Source: CAD feature listing. Evaluate the final solid. Frame: model axes, mm. Face numbers are marked on the shaded views. A direction names the side the tool comes from. Give positions to 0.01 mm unless a question says otherwise; leave off trailing zeros. Order: outer loops, then holes, each group sorted by start corner. A loop starts at its lowest first (then second) coordinate and runs counter-clockwise, first axis right, second up. Notation, with made-up numbers: M 48,60.25 L 63,60.25 A25 cw 63,89.25 Z; hole C 65.25,-38.75 d11. An arc over 180 degrees is marked long. Answer in a Markdown table with one row per item. Add a question column.
(1) Pin query (flat end, axial travel): P1, Ø1.5, axis at x = 76.5, z = -47.5, coming from the +Y side; P2, Ø22.5, axis at x = 24.5, y = 1.5, coming from the +Z side; P3, Ø10, axis at y = 1, z = -11.5, coming from the +X side. Return the tip coordinate at first contact, or that it passes through.
(2) Section query C-C, the plane z = -19.5. Return loops of the section in (x, y), plus the area to 3 significant figures.
(3) Section query B-B, the plane x = -25.5. Return loops of the section in (y, z).
(4) Material intervals for line 1 along Z through (x, y) = (7, 19.4); line 2 along X through (y, z) = (19.45, -47); line 3 along Z through (x, y) = (-53, 16), sorted ascending.
(5) Set-up query: the marked faces 1 and 2. Return all of +Z, -Z, +X, -X, +Y, -Y with unobstructed straight access to the full face (end or side cutting, diameter ignored); none if empty.
(6) Section query A-A, the plane y = -16.5. Return loops of the section in (x, z).
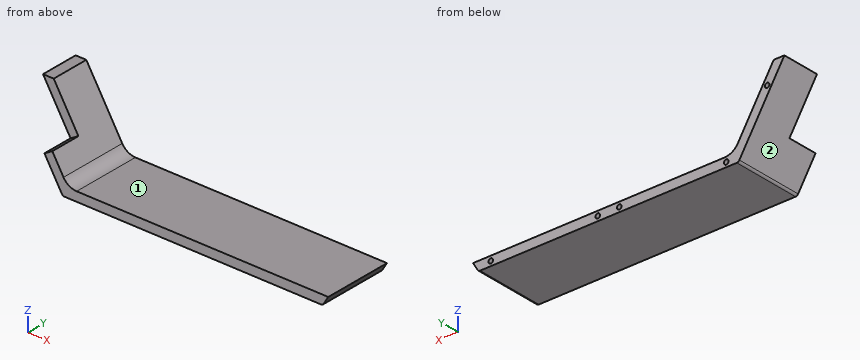
from build123d import *

# Parameters (mm, degrees)
BOSS_EXTRUDE1_DEPTH = 22.5
SKETCH2_R           = 1.5
CUT_EXTRUDE1_DEPTH  = 5
FILLET1_R           = 2
SKETCH3_W           = 35
SKETCH3_H           = 20
CUT_EXTRUDE2_DEPTH  = 10
SKETCH6_W           = 44
SKETCH6_H           = 45
CUT_EXTRUDE3_DEPTH  = 128.401923062
FILLET2_R           = 10


with BuildPart() as part:
    # Sketch1 → Boss-Extrude1 (new, symmetric)
    with BuildSketch(Plane(origin=(0, 0, 0), x_dir=(1, 0, 0), z_dir=(0, 1, 0))):
        Polygon((-115, 0), (-85, 50), (85, 50), (115, 0), (108, 0), (81.6, 44), (-81.6, 44), (-108, 0), align=None)
    extrude(amount=BOSS_EXTRUDE1_DEPTH, both=True)

    # Sketch2 → Cut-Extrude1 (cut)
    with BuildSketch(Plane(origin=(0, 22.5, 0), x_dir=(1, 0, 0), z_dir=(0, 1, 0))):
        with Locations(Location((-103.701428863, 13, 0), (0, 0, 270))):
            Circle(SKETCH2_R)
        with Locations(Location((-77, 47, 0), (0, 0, 270))):
            Circle(SKETCH2_R)
        with Locations(Location((-7, 47, 0), (0, 0, 270))):
            Circle(SKETCH2_R)
        with Locations(Location((7, 47, 0), (0, 0, 90))):
            Circle(SKETCH2_R)
        with Locations(Location((77, 47, 0), (0, 0, 90))):
            Circle(SKETCH2_R)
        with Locations(Location((103.701428863, 13, 0), (0, 0, 90))):
            Circle(SKETCH2_R)
    extrude(amount=-CUT_EXTRUDE1_DEPTH, mode=Mode.SUBTRACT)

    # Fillet1
    fillet1_edges = [part.edges().sort_by_distance(p)[0] for p in [
        (-85, 0, -50),
        (85, 0, -50),
    ]]
    fillet(fillet1_edges, radius=FILLET1_R)

    # Sketch3 → Cut-Extrude2 (cut)
    with BuildSketch(Plane(origin=(-84.558823529, 0, -50.735294118), x_dir=(-0.5144957554275263, 0, 0.8574929257125444), z_dir=(-0.8574929257125444, 0, -0.5144957554275263))):
        with Locations((41.667011874, -12.5)):
            Rectangle(SKETCH3_W, SKETCH3_H)
    extrude(amount=-CUT_EXTRUDE2_DEPTH, mode=Mode.SUBTRACT)

    # Sketch6 → Cut-Extrude3 (cut, through all)
    with BuildSketch(Plane(origin=(0, 0, 0), x_dir=(0, 0, -1), z_dir=(1, 0, 0))):
        with Locations((22, 0)):
            Rectangle(SKETCH6_W, SKETCH6_H)
    extrude(amount=CUT_EXTRUDE3_DEPTH, mode=Mode.SUBTRACT)

    # Fillet2
    fillet2_edges = [part.edges().sort_by_distance(p)[0] for p in [
        (-81.6, 0, -44),
    ]]
    fillet(fillet2_edges, radius=FILLET2_R)


solid = part.part
Values follow:
| question | item | result |
|---|---|---|
| 1 | P1 | stops at y = 17.5 |
| 1 | P2 | stops at z = -44 |
| 1 | P3 | stops at x = -98.1 |
| 2 | outline | M -103.3,-2.5 L -96.3,-2.5 L -96.3,22.5 L -103.3,22.5 Z |
| 2 | area | 175 mm² |
| 3 | outline | M -22.5,-50 L 22.5,-50 L 22.5,-44 L -22.5,-44 Z |
| 4 | line 1 | z = -50 to -48.5, -45.5 to -44 |
| 4 | line 2 | x = -86.8 to -78.5, -75.5 to -8.5, -5.5 to 5.5, 8.5 to 75.5, 78.5 to 86.8 |
| 4 | line 3 | z = -50 to -44 |
| 5 | face 1 | +Z, +X, +Y, -Y |
| 5 | face 2 | -Z, -X, +Y, -Y |
| 6 | outline | M -96.99,-30.01 L -85.58,-49.03 A2 ccw -83.87,-50 L 83.87,-50 A2 ccw 85.58,-49.03 L 88.6,-44 L -75.94,-44 A10 cw -84.51,-39.14 L -91.85,-26.92 Z |
